The model under review builds one solid part; all positions refer to its coordinate system, in mm. Face numbers are marked on the shaded views. A direction names the side the tool comes from. Coordinates: 2 decimals unless noted, no trailing zeros. Loops run counter-clockwise (first coordinate to the right, second up) from the corner with the lowest first, then second, coordinate; pieces in that order, holes last. Notation, with made-up numbers: M 5,24 L 15,24 A31 cw 15,61 Z; hole C -28,53 d5. An arc over 180 degrees is marked long. Use CSV: the item, a comma, the result in double quotes. Start each with the question number.
1. Add section C-C, the plane y = -53.5. Write out the cut boundary in (x, z) (3 decimals).
2. Add section D-D, the plane z = 3.81. Write out the cut boundary in (x, y) (3 decimals), then the cut area to 3 significant figures.
3. Add section B-B, the plane z = -11. Write out the cut boundary in (x, y).
4. Tool access review of the marked faces 1, 2, 3, 4 and 5: name each direction out of +Z, -Z, +X, -X, +Y, -Y from which nothing blocks a thin tool from reaching the whole face with its end or side.
5. For L1, parallel to Z at x = 0.5, y = -54; L2, parallel to Y at x = 0, z = 9.7; L3, parallel to Z at x = 13, y = -10, list the stretches that pass through material, from the lowest coordinate up.
6. Clearance check with flat-ended pins moving along their axes: P1, Ø9, axis at y = -10.16, z = -19.05, coming from the +X side; P2, Ø11.5, axis at y = -56.5, z = 17, coming from the +X side (3 decimals); P3, Ø2, axis at y = -55, z = 18.5, coming from the -X side (3 decimals); P4, Ø2.5, axis at x = 12.5, z = -9.5, coming from the -Y side. State where each tip first meets the part, or that it passes through.
7. Add section A-A, the plane x = 0. State how many separate pieces and enclosed holes the cut face has, then the cut area to 3 significant figures.
8. Draft analysis for pull direction Z (two halves, no side actions). For the marked faces 6, 7 and 8, state which applies: +Z half, -Z half, draft (parallel to the pull), parting line (faces both ways), or undercut.
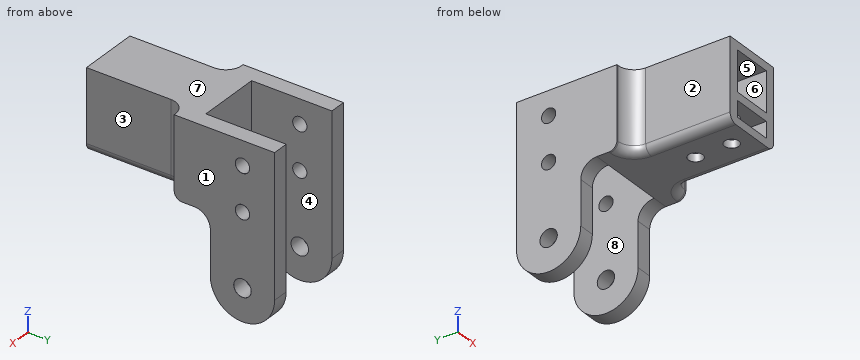
from build123d import *

# Parameters (mm, degrees)
BOSS_EXTRUDE1_DEPTH            = 25.4
SKETCH2_W                      = 12.7
SKETCH2_H                      = 12.7
SKETCH2_H_2                    = 5.08
CUT_EXTRUDE1_DEPTH             = 31.75
M4_CLEARANCE_HOLE4_D           = 4.5
M4_CLEARANCE_HOLE4_DEPTH       = 10.16
M4_CLEARANCE_HOLE4_CSINK_D     = 4.55
M4_CLEARANCE_HOLE4_CSINK_ANGLE = 100
M4_CLEARANCE_HOLE4_TIP         = 1.351936393
SKETCH6_W                      = 5.08
SKETCH6_H                      = 20.32
BOSS_EXTRUDE2_DEPTH            = 19.05
BOSS_EXTRUDE3_DEPTH            = 5.08
BOSS_EXTRUDE4_DEPTH            = 5.08
M4_CLEARANCE_HOLE5_D           = 4.5
M4_CLEARANCE_HOLE5_DEPTH       = 30.226
M4_CLEARANCE_HOLE5_CSINK_D     = 4.55
M4_CLEARANCE_HOLE5_CSINK_ANGLE = 100
M4_CLEARANCE_HOLE5_TIP         = 1.351936393
M5_CLEARANCE_HOLE1_D           = 5.5
M5_CLEARANCE_HOLE1_DEPTH       = 30.226
M5_CLEARANCE_HOLE1_CSINK_D     = 5.55
M5_CLEARANCE_HOLE1_CSINK_ANGLE = 100
M5_CLEARANCE_HOLE1_TIP         = 1.652366702
FILLET1_R                      = 5.08
FILLET2_R                      = 2.54


with BuildPart() as part:
    # Sketch1 → Boss-Extrude1 (new body)
    with BuildSketch(Plane.XY):
        Polygon((-15.113, 0), (-10.033, 0), (-10.033, -25.4), (10.033, -25.4), (10.033, 0), (15.113, 0), (15.113, -31.75), (9.525, -31.75), (9.525, -63.5), (-9.525, -63.5), (-9.525, -31.75), (-15.113, -31.75), align=None)
    extrude(amount=BOSS_EXTRUDE1_DEPTH)

    # Sketch2 → Cut-Extrude1 (cut)
    with BuildSketch(Plane.XZ.offset(63.5)):
        with Locations((0, 16.51)):
            Rectangle(SKETCH2_W, SKETCH2_H)
        with Locations((0, 5.08)):
            Rectangle(SKETCH2_W, SKETCH2_H_2)
    extrude(amount=-CUT_EXTRUDE1_DEPTH, mode=Mode.SUBTRACT)

    # M4 Clearance Hole4
    with Locations(Plane(origin=(0, 0, 0), x_dir=(-1, 0, 0), z_dir=(0, 0, -1))):
        with Locations((0, -57.15), (0, -45.72)):
            CounterSinkHole(M4_CLEARANCE_HOLE4_D / 2, M4_CLEARANCE_HOLE4_CSINK_D / 2, depth=M4_CLEARANCE_HOLE4_DEPTH, counter_sink_angle=M4_CLEARANCE_HOLE4_CSINK_ANGLE)
            with Locations((0, 0, -(M4_CLEARANCE_HOLE4_DEPTH + M4_CLEARANCE_HOLE4_TIP / 2))):  # 118° drill point
                Cone(0, M4_CLEARANCE_HOLE4_D / 2, M4_CLEARANCE_HOLE4_TIP, mode=Mode.SUBTRACT)

    # Sketch6 → Boss-Extrude2 (add)
    with BuildSketch(Plane(origin=(0, 0, 0), x_dir=(-1, 0, 0), z_dir=(0, 0, -1))):
        with Locations((-12.573, -10.16)):
            Rectangle(SKETCH6_W, SKETCH6_H)
        with Locations((12.573, -10.16)):
            Rectangle(SKETCH6_W, SKETCH6_H)
    extrude(amount=BOSS_EXTRUDE2_DEPTH)

    # Sketch7 → Boss-Extrude3 (add)
    with BuildSketch(Plane(origin=(15.113, 0, 0), x_dir=(0, 0, -1), z_dir=(1, 0, 0))):
        with BuildLine():
            Line((19.05, -20.32), (19.05, 0))
            ThreePointArc((19.05, 0), (29.21, -10.16), (19.05, -20.32))
        make_face()
    extrude(amount=-BOSS_EXTRUDE3_DEPTH)

    # Sketch8 → Boss-Extrude4 (add)
    with BuildSketch(Plane.ZY.offset(15.113)):
        with BuildLine():
            Line((-19.05, -20.32), (-19.05, 0))
            ThreePointArc((-19.05, 0), (-29.21, -10.16), (-19.05, -20.32))
        make_face()
    extrude(amount=-BOSS_EXTRUDE4_DEPTH)

    # M4 Clearance Hole5
    with Locations(Plane(origin=(15.113, 0, 0), x_dir=(0, 0, -1), z_dir=(1, 0, 0))):
        with Locations((-17.78, -10.16), (-3.81, -10.16)):
            CounterSinkHole(M4_CLEARANCE_HOLE5_D / 2, M4_CLEARANCE_HOLE5_CSINK_D / 2, depth=M4_CLEARANCE_HOLE5_DEPTH, counter_sink_angle=M4_CLEARANCE_HOLE5_CSINK_ANGLE)
            with Locations((0, 0, -(M4_CLEARANCE_HOLE5_DEPTH + M4_CLEARANCE_HOLE5_TIP / 2))):  # 118° drill point
                Cone(0, M4_CLEARANCE_HOLE5_D / 2, M4_CLEARANCE_HOLE5_TIP, mode=Mode.SUBTRACT)

    # M5 Clearance Hole1
    with Locations(Plane(origin=(15.113, 0, 0), x_dir=(0, 0, -1), z_dir=(1, 0, 0))):
        with Locations((19.05, -10.16)):
            CounterSinkHole(M5_CLEARANCE_HOLE1_D / 2, M5_CLEARANCE_HOLE1_CSINK_D / 2, depth=M5_CLEARANCE_HOLE1_DEPTH, counter_sink_angle=M5_CLEARANCE_HOLE1_CSINK_ANGLE)
            with Locations((0, 0, -(M5_CLEARANCE_HOLE1_DEPTH + M5_CLEARANCE_HOLE1_TIP / 2))):  # 118° drill point
                Cone(0, M5_CLEARANCE_HOLE1_D / 2, M5_CLEARANCE_HOLE1_TIP, mode=Mode.SUBTRACT)

    # Fillet1
    fillet1_edges = [part.edges().sort_by_distance(p)[0] for p in [
        (12.573, -20.32, 0),
        (-12.573, -20.32, 0),
        (-9.525, -31.75, 12.7),
        (9.525, -31.75, 12.7),
    ]]
    fillet(fillet1_edges, radius=FILLET1_R)

    # Fillet2
    fillet2_edges = [part.edges().sort_by_distance(p)[0] for p in [
        (9.525, -50.165, 0),
        (14.859, -31.75, 0),
        (-9.525, -50.165, 0),
        (-14.859, -31.75, 0),
        (-11.012897552, -33.237897552, 0),
        (11.012897552, -33.237897552, 0),
    ]]
    fillet(fillet2_edges, radius=FILLET2_R)


solid = part.part
Computed:
1,outline,"M -9.525,2.54 A2.54 ccw -6.985,0 L 6.985,0 A2.54 ccw 9.525,2.54 L 9.525,25.4 L -9.525,25.4 Z; hole M -6.35,2.54 L 6.35,2.54 L 6.35,7.62 L -6.35,7.62 Z; hole M -6.35,10.16 L 6.35,10.16 L 6.35,22.86 L -6.35,22.86 Z"
2,outline,"M -15.113,-31.75 L -14.605,-31.75 A5.08 cw -9.525,-36.83 L -9.525,-63.5 L -6.35,-63.5 L -6.35,-31.75 L 6.35,-31.75 L 6.35,-63.5 L 9.525,-63.5 L 9.525,-36.83 A5.08 cw 14.605,-31.75 L 15.113,-31.75 L 15.113,-12.435 L 15.092,-12.41 L 10.033,-12.41 L 10.033,-25.4 L -10.033,-25.4 L -10.033,-12.41 L -15.113,-12.41 Z; M -15.113,-7.91 L -10.033,-7.91 L -10.033,0 L -15.113,0 Z; M 10.033,-7.91 L 15.092,-7.91 L 15.113,-7.885 L 15.113,0 L 10.033,0 Z"
2,area,"617 mm^2"
3,outline,"M -15.11,-20.32 L -10.03,-20.32 L -10.03,0 L -15.11,0 Z; M 10.03,-20.32 L 15.11,-20.32 L 15.11,0 L 10.03,0 Z"
4,face 1,"+Z, -Z, +X, +Y, -Y"
4,face 2,"+Z, -Z, -X, -Y"
4,face 3,"+Z, -Z, +X, -Y"
4,face 4,"+Z, -Z, +Y"
4,face 5,"-Y"
5,L1,"z = 0 to 2.54, 7.62 to 10.16, 22.86 to 25.4"
5,L2,"y = -63.5 to -59.4, -54.9 to -47.97, -43.47 to -25.4"
5,L3,"z = -29.21 to -21.8, -16.3 to 1.57, 6.05 to 15.54, 20.02 to 25.4"
6,P1,"stops at x = 15.11"
6,P2,"stops at x = 9.525"
6,P3,"stops at x = -9.525"
6,P4,"stops at y = -20.32"
7,separate pieces,"5"
7,enclosed holes,"0"
7,area,"358 mm^2"
8,face 6,"undercut"
8,face 7,"+Z half"
8,face 8,"draft"
